The listing builds one solid part. Answer for the finished solid, in the listing's coordinates (mm). Face numbers are marked on the shaded views. A direction names the side the tool comes from. Round coordinates to 2 decimals unless told otherwise and drop trailing zeros. Loops run counter-clockwise (first coordinate to the right, second up) from the corner with the lowest first, then second, coordinate; pieces in that order, holes last. Notation, with made-up numbers: M 71,-29 L 114,-29 A13 cw 114,-11 Z; hole C 30.5,5 d1. An arc over 180 degrees is marked long. Answer as a JSON object with one key per item and string values.
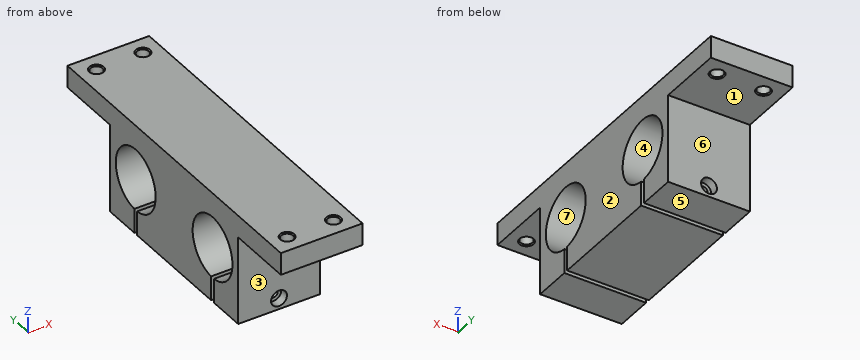
```python
from build123d import *

# Parameters (mm, degrees)
F1_DEPTH  = 37
F2_R      = 2
F3_DEPTH  = 30
F4_R      = 3.6
F5_DEPTH  = 4
F6_R      = 2
F7_DEPTH  = 30
F8_R      = 3.6
F9_DEPTH  = 4
F10_R     = 2.75
F11_DEPTH = 50.001
F12_SIZE  = 0.5


with BuildPart() as f1:
    # F0 (on Right) → F1 (new body)
    with BuildSketch(Plane.YZ):
        with BuildLine():
            Line((-45, 0), (-45, -40))
            Line((-45, -40), (-28, -40))
            Line((-28, -40), (-28, -28.9642400438))
            ThreePointArc((-28, -28.9642400438), (-27, -1), (-26, -28.9642400438))
            Line((-26, -28.9642400438), (-26, -40))
            Line((-26, -40), (26, -40))
            Line((26, -40), (26, -28.9642400438))
            ThreePointArc((26, -28.9642400438), (27, -1), (28, -28.9642400438))
            Line((28, -28.9642400438), (28, -40))
            Line((28, -40), (45, -40))
            Line((45, -40), (45, 0))
            Line((45, 0), (75, 0))
            Line((75, 0), (75, 10))
            Line((75, 10), (-75, 10))
            Line((-75, 10), (-75, 0))
            Line((-75, 0), (-45, 0))
        make_face()
    extrude(amount=F1_DEPTH)

    # F2 (on face) → F3 (cut)
    with BuildSketch(Plane.XZ.offset(45)):
        with Locations((18.5, -35)):
            Circle(F2_R)
    extrude(amount=-F3_DEPTH, mode=Mode.SUBTRACT)

    # F4 (on face) → F5 (cut)
    with BuildSketch(Plane.XZ.offset(45)):
        with Locations((18.5, -35)):
            Circle(F4_R)
    extrude(amount=-F5_DEPTH, mode=Mode.SUBTRACT)

    # F6 (on face) → F7 (cut)
    with BuildSketch(Plane(origin=(0, 45, 0), x_dir=(-1, 0, 0), z_dir=(0, 1, 0))):
        with Locations((-18.5, -35)):
            Circle(F6_R)
    extrude(amount=-F7_DEPTH, mode=Mode.SUBTRACT)

    # F8 (on face) → F9 (cut)
    with BuildSketch(Plane(origin=(0, 45, 0), x_dir=(-1, 0, 0), z_dir=(0, 1, 0))):
        with Locations((-18.5, -35)):
            Circle(F8_R)
    extrude(amount=-F9_DEPTH, mode=Mode.SUBTRACT)

    # F10 (on face) → F11 (cut, through all)
    with BuildSketch(Plane.XY.offset(10)):
        with Locations((29, 67)):
            Circle(F10_R)
        with Locations((8, 67)):
            Circle(F10_R)
        with Locations((8, -67)):
            Circle(F10_R)
        with Locations((29, -67)):
            Circle(F10_R)
    extrude(amount=-F11_DEPTH, mode=Mode.SUBTRACT)

    # F12
    f12_edges = [f1.edges().sort_by_distance(p)[0] for p in [
        (5.25, 67, 10),
        (10.75, 67, 5),
        (5.25, 67, 0),
        (26.25, 67, 10),
        (31.75, 67, 5),
        (26.25, 67, 0),
        (5.25, -67, 10),
        (10.75, -67, 5),
        (5.25, -67, 0),
        (26.25, -67, 10),
        (31.75, -67, 5),
        (26.25, -67, 0),
    ]]
    chamfer(f12_edges, length=F12_SIZE)


solid = f1.part
```
Item 1: Determine the mould class of the marked faces 4, 5, 6 and 7 for opening direction Z: released by +Z, released by -Z, zero draft, split by the parting line, or undercut.
Values follow:
{"face 4": "undercut", "face 5": "released by -Z", "face 6": "zero draft", "face 7": "undercut"}
Item 2: The part is cut by section D-D (x = 34). Give the vertices of the cut face in (y, z).
Values follow:
{"outline": "M -75,0 L -45,0 L -45,-40 L -28,-40 L -28,-28.96 A14 cw long -26,-28.96 L -26,-40 L 26,-40 L 26,-28.96 A14 cw long 28,-28.96 L 28,-40 L 45,-40 L 45,0 L 75,0 L 75,10 L -75,10 Z"}
Item 3: Straight lines are drawn through the part: line 1 (Y direction, x = 29, z = -14.5); line 2 (Y direction, x = 8, z = 5.75); line 3 (Z direction, x = 12.5, y = 62.5). For each, find the intervals that lie inside material, in ascending order.
Values follow:
{"line 1": "-45 to -40.99, -13.01 to 13.01, 40.99 to 45", "line 2": "-75 to -69.75, -64.25 to 64.25, 69.75 to 75", "line 3": "0 to 10"}
Item 4: Which of the six approach directions +Z, -Z, +X, -X, +Y, -Y give full straight-line access (tool end or side, diameter ignored) to the marked faces 1, 2 and 3?
Values follow:
{"face 1": "-Z, +X, -X, +Y", "face 2": "+Z, -Z, +X, +Y, -Y", "face 3": "-Z, +X, -X, -Y"}
Item 5: Flat-ended cylindrical pins translate along their axes: P1, Ø2, axis at x = 17, z = -36, coming from the +Y side; P2, Ø3.5, axis at x = 18.5, z = -35, coming from the -Y side; P3, Ø3.5, axis at x = 18, z = -32.5, coming from the +Y side. Find the tip coordinate at first contact, or state that the pin passes through.
Values follow:
{"P1": "y = 41", "P2": "y = -15", "P3": "y = 45"}
Item 6: The part is cut by section B-B (y = 67). Give the vertices of the cut face in (x, z).
Values follow:
{"outline": "M 0,0 L 4.75,0 L 5.25,0.5 L 5.25,9.5 L 4.75,10 L 0,10 Z; M 10.75,0.5 L 11.25,0 L 25.75,0 L 26.25,0.5 L 26.25,9.5 L 25.75,10 L 11.25,10 L 10.75,9.5 Z; M 31.75,0.5 L 32.25,0 L 37,0 L 37,10 L 32.25,10 L 31.75,9.5 Z"}
Item 7: The part is cut by section A-A (x = 8). Give the number of separate pieces and of enclosed holes in the cut face, then the cut area to 3 significant figures.
Values follow:
{"separate pieces": "3", "enclosed holes": "0", "area": "3,710 mm^2"}
Item 8: The part is cut by section C-C (z = -18). Give the vertices of the cut face in (x, y).
Values follow:
{"outline": "M 0,-45 L 37,-45 L 37,-40.67 L 0,-40.67 Z; M 0,-13.33 L 37,-13.33 L 37,13.33 L 0,13.33 Z; M 0,40.67 L 37,40.67 L 37,45 L 0,45 Z"}
